Read the model definition and answer for the solid it produces. Units are mm, in the model's axes. Give positions to 0.01 mm unless a question says otherwise; leave off trailing zeros. Order: outer loops, then holes, each group sorted by start corner. A loop starts at its lowest first (then second) coordinate and runs counter-clockwise, first axis right, second up. Notation, with made-up numbers: (70.25, 20) -> (76.25, 20) arc R29 cw to (76.25, 48) -> close; hole circle Ø9 at (70.5, -36.5). An arc over 180 degrees is marked (long way). One line per question, with ' | ' between items. Start each with the question number.
```python
from build123d import *

# Parameters (mm, degrees)
CYLINDER017_R     = 1.4
CYLINDER017_DEPTH = 2
CYLINDER018_R     = 1.4
CYLINDER018_DEPTH = 2
BOX008_W          = 16
BOX008_H          = 42
BOX008_DEPTH      = 1


with BuildPart() as zylinder017:
    # Cylinder017 → Cylinder017 (new body)
    with BuildSketch(Plane(origin=(16.5, 10, -29.5), x_dir=(1, 0, 0), z_dir=(0, 0, 1))):
        Circle(CYLINDER017_R)
    extrude(amount=CYLINDER017_DEPTH)


with BuildPart() as zylinder018:
    # Cylinder018 → Cylinder018 (new body)
    with BuildSketch(Plane(origin=(16.5, -10, -29.5), x_dir=(1, 0, 0), z_dir=(0, 0, 1))):
        Circle(CYLINDER018_R)
    extrude(amount=CYLINDER018_DEPTH)


with BuildPart() as fusion007:
    # Box008 → Box008 (new body)
    with BuildSketch(Plane(origin=(8.5, -21, -27.5), x_dir=(1, 0, 0), z_dir=(0, 0, 1))):
        with Locations((8, 21)):
            Rectangle(BOX008_W, BOX008_H)
    extrude(amount=BOX008_DEPTH)

    # Fusion007: union Zylinder017, Zylinder018
    add(zylinder017.part)
    add(zylinder018.part)


with BuildPart() as fusion007_1:
    # Fusion007 placement: moved
    add(fusion007.part.moved(Location((-34.5, 0, 0.5))))


solid = fusion007_1.part
```
Q1. A cutting plane is placed at D-D, the plane x = -16. Determine the outline of the cut face in (y, z), then the cut area to 3 significant figures.
Q2. Determine the mould class of faces 1 (the flat face through (-18, -10, -29)), 2 (the cylindrical face through (-18.303, -11.367, -28.014)), 3 (the cylindrical face through (-19.03, 10.95, -28.01)), 4 (the flat face through (-18.1, -21, -26.5)) for opening direction Y: pulls with the +Y half, pulls with the -Y half, needs draft (parallel to the pull), parting line crosses it, or undercut.
Q3. A cutting plane is placed at B-B, the plane z = -27.95. Determine the outline of the cut face in (x, y).
Q4. Find the intervals of material crossed by line 1 (Z direction, x = -18.25, y = -6); line 2 (Y direction, x = -17.5, z = -27.65); line 3 (Y direction, x = -17.75, z = -28.5), in increasing order.
Q5. A cutting plane is placed at C-C, the plane y = 10. Determine the outline of the cut face in (x, z), then the cut area to 3 significant figures.
Q6. Given P1, Ø5, axis at x = -22, y = 10, coming from the -Z side, flat-ended and moving along its own axis, determine where the tip first touches the part or whether it passes through.
Q7. A cutting plane is placed at A-A, the plane x = -18. Determine the outline of the cut face in (y, z).
Geometry results:
1) outline: (-21, -27) -> (21, -27) -> (21, -26) -> (-21, -26) -> close | area: 42.0 mm²
2) face 1: needs draft | face 2: undercut | face 3: undercut | face 4: pulls with the -Y half
3) outline: circle Ø2.8 at (-18, -10); circle Ø2.8 at (-18, 10)
4) line 1: -27 to -26 | line 2: -11.31 to -8.69, 8.69 to 11.31 | line 3: -11.38 to -8.62, 8.62 to 11.38
5) outline: (-26, -27) -> (-19.4, -27) -> (-19.4, -29) -> (-16.6, -29) -> (-16.6, -27) -> (-10, -27) -> (-10, -26) -> (-26, -26) -> close | area: 21.6 mm²
6) P1: z = -27
7) outline: (-21, -27) -> (-11.4, -27) -> (-11.4, -29) -> (-8.6, -29) -> (-8.6, -27) -> (8.6, -27) -> (8.6, -29) -> (11.4, -29) -> (11.4, -27) -> (21, -27) -> (21, -26) -> (-21, -26) -> close
